from build123d import *

# Parameters (mm, degrees)
SKETCH1_W             = 30.5
SKETCH1_H             = 30.5
BOSS_EXTRUDE1_DEPTH   = 3
SKETCH2_W             = 10
SKETCH2_H             = 60
BOSS_EXTRUDE2_DEPTH   = 3
BOSS_EXTRUDE3_DEPTH   = 3
F_3_0MM_DOWEL_HOLE1_D = 3
FILLET1_R             = 4
FILLET2_R             = 10
SKETCH6_R             = 3
CUT_EXTRUDE1_DEPTH    = 3
F_4_0MM_DOWEL_HOLE1_D = 4
F_4_0MM_DOWEL_HOLE2_D = 4


with BuildPart() as part:
    # Sketch1 → Boss-Extrude1 (new body)
    with BuildSketch(Plane.XY):
        with Locations((15.25, 15.25)):
            Rectangle(SKETCH1_W, SKETCH1_H)
    extrude(amount=BOSS_EXTRUDE1_DEPTH)

    # Sketch2 → Boss-Extrude2 (add)
    with BuildSketch(Plane.XZ):
        with Locations((15.25, 33)):
            Rectangle(SKETCH2_W, SKETCH2_H)
    extrude(amount=-BOSS_EXTRUDE2_DEPTH)

    # Sketch3 → Boss-Extrude3 (add)
    with BuildSketch(Plane.XZ):
        Polygon((22.565242881, 50.684757119), (13.584450202, 41.70396444), (-14.699821045, 69.988235687), (1.563634922, 86.251691655), (15.705770546, 72.109556031), (27.726585826, 84.130371311), (41.86872145, 69.988235687), align=None)
    extrude(amount=-BOSS_EXTRUDE3_DEPTH)

    # Ø3.0mm Dowel Hole1 (through all)
    with Locations(Plane.XY.offset(3)):
        with Locations((4, 9.8), (26.8, 25.5)):
            Hole(F_3_0MM_DOWEL_HOLE1_D / 2)

    # Fillet1
    fillet1_edges = [part.edges().sort_by_distance(p)[0] for p in [
        (10.25, 1.5, 3),
        (15.25, 3, 3),
        (20.25, 1.5, 3),
    ]]
    fillet(fillet1_edges, radius=FILLET1_R)

    # Fillet2
    fillet2_edges = [part.edges().sort_by_distance(p)[0] for p in [
        (20.25, 1.5, 48.369514237),
        (10.25, 1.5, 45.038414642),
    ]]
    fillet(fillet2_edges, radius=FILLET2_R)

    # Sketch6 → Cut-Extrude1 (cut)
    with BuildSketch(Plane(origin=(0, 3, 0), x_dir=(1, 0, 0), z_dir=(0, 1, 0))):
        with Locations(Location((15.25, -57, 0), (0, 0, 270))):
            Circle(SKETCH6_R)
    extrude(amount=-CUT_EXTRUDE1_DEPTH, mode=Mode.SUBTRACT)

    # Ø4.0mm Dowel Hole1 (through all)
    with Locations(Plane(origin=(0, 3, 0), x_dir=(1, 0, 0), z_dir=(0, 1, 0))):
        with Locations((0.14942136, -70.695342468)):
            Hole(F_4_0MM_DOWEL_HOLE1_D / 2)

    # Ø4.0mm Dowel Hole2 (through all)
    with Locations(Plane(origin=(0, 3, 0), x_dir=(1, 0, 0), z_dir=(0, 1, 0))):
        with Locations((29.140799389, -68.574022125)):
            Hole(F_4_0MM_DOWEL_HOLE2_D / 2)


solid = part.part
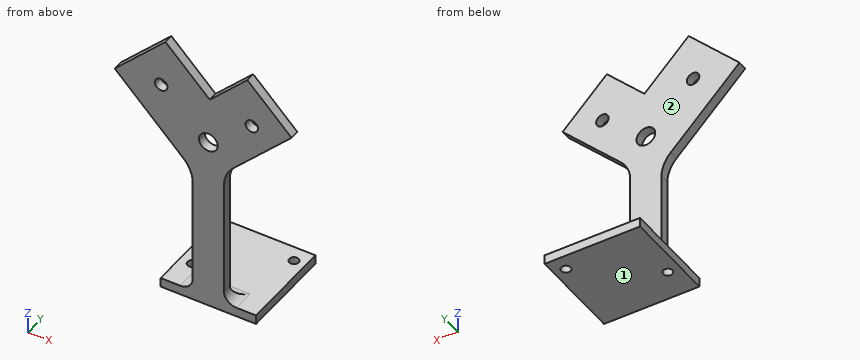
The model under review builds one solid part; all positions refer to its coordinate system, in mm. Face numbers are marked on the shaded views. A direction names the side the tool comes from. Coordinates: 2 decimals unless noted, no trailing zeros. Write each loop counter-clockwise with the first axis right and the second up, starting at its lowest first coordinate (ties: lowest second). Pieces come first, ordered by that corner, then holes. Notation, with made-up numbers: (85.5, 37) - (95.5, 37) arc R11 ccw to (95.5, 44) - close; hole circle Ø10 at (-9.75, 46). An arc over 180 degrees is marked (long way). Answer as a JSON object with one key per item and string values. Group by question number.
1. To check wall thickness, follow probe 1 along Y at (x, z) = (26.8, 0.75); probe 2 along Z at (x, y) = (29, 14.5). State the ranges of each line that lie inside material, in increasing order.
2. Add section D-D (y = 15). Give the boundary of the cut face in (x, z).
3. Clearance check with flat-ended pins moving along their axes: pin 1 Ø1.5 at (y, z) = (2, 19.5) entering from +X; pin 2 Ø9.5 at (x, z) = (15.25, 57) entering from +Y; pin 3 Ø3.5 at (x, y) = (4, 9.8) entering from +Z. State where each tip first meets the part, or that it passes through.
4. Add section A-A (y = 25.5). Give the boundary of the cut face in (x, z), plus the area to 3 significant figures.
5. Add section B-B (z = 57). Give the boundary of the cut face in (x, y), plus the area to 3 significant figures.
6. Add section C-C (x = 4). Give the boundary of the cut face in (y, z).
7. Machinability: for the marked faces 1 and 2, which of the approach directions +Z, -Z, +X, -X, +Y, -Y give a long, thin tool a straight path to every point of the face, cutting with its end or side? Answer none if there is none.
Findings:
{
 "1": {"probe 1": "0 to 24, 27 to 30.5", "probe 2": "0 to 3"},
 "2": {"outline": "(0, 0) - (30.5, 0) - (30.5, 3) - (0, 3) - close"},
 "3": {"pin 1": "x = 20.25", "pin 2": "y = 3", "pin 3": "z = 3"},
 "4": {"outline": "(0, 0) - (25.3, 0) - (25.3, 3) - (0, 3) - close; (28.3, 0) - (30.5, 0) - (30.5, 3) - (28.3, 3) - close", "area": "82.5 mm²"},
 "5": {"outline": "(-1.71, 0) - (12.25, 0) - (12.25, 3) - (-1.71, 3) - close; (18.25, 0) - (28.88, 0) - (28.88, 3) - (18.25, 3) - close", "area": "73.8 mm²"},
 "6": {"outline": "(0, 0) - (8.3, 0) - (8.3, 3) - (0, 3) - close; (0, 51.29) - (3, 51.29) - (3, 83.82) - (0, 83.82) - close; (11.3, 0) - (30.5, 0) - (30.5, 3) - (11.3, 3) - close"},
 "7": {"face 1": "-Z, +X, -X, +Y, -Y", "face 2": "+Z, +X, -X, +Y"}
}
